```python
from build123d import *

# Parameters (mm, degrees)
BOSS_EXTRUDE1_DEPTH      = 25
BOSS_EXTRUDE1_DEPTH_BACK = 25
SKETCH1_W                = 70
SKETCH1_H                = 10
BOSS_EXTRUDE2_DEPTH      = 10
BOSS_EXTRUDE2_DEPTH_BACK = 10
CUT_EXTRUDE1_DEPTH       = 19
CUT_EXTRUDE1_DEPTH_BACK  = 16
SKETCH3_R                = 3.5


with BuildPart() as part:
    # Sketch1 → Boss-Extrude1 (new, two sides: drawn at the far end of the back side and taken through both)
    with BuildSketch(Plane(origin=(0, 0, 0), x_dir=(1, 0, 0), z_dir=(0, 1, 0)).offset(-BOSS_EXTRUDE1_DEPTH_BACK)):
        Rectangle(SKETCH1_W, SKETCH1_H)
    extrude(amount=BOSS_EXTRUDE1_DEPTH + BOSS_EXTRUDE1_DEPTH_BACK)

    # Sketch2 → Boss-Extrude2 (add, two sides: drawn at the far end of the back side and taken through both)
    with BuildSketch(Plane(origin=(0, 0, 0), x_dir=(1, 0, 0), z_dir=(0, 1, 0)).offset(-BOSS_EXTRUDE2_DEPTH_BACK)):
        with BuildLine():
            Line((-75, 5), (-35, 5))
            Line((-35, 5), (-35, -5))
            Line((-35, -5), (-75, -5))
            ThreePointArc((-75, -5), (-80, 0), (-75, 5))
        make_face()
    extrude(amount=BOSS_EXTRUDE2_DEPTH + BOSS_EXTRUDE2_DEPTH_BACK)

    # Sketch3 → Cut-Extrude1 (cut, two sides: drawn at the far end of the back side and taken through both)
    with BuildSketch(Plane(origin=(0, 0, 0), x_dir=(1, 0, 0), z_dir=(0, 1, 0)).offset(-CUT_EXTRUDE1_DEPTH_BACK)):
        with Locations(Location((-75.333177097, 0, 0), (0, 0, 270))):
            Circle(SKETCH3_R)
        with Locations(Location((-55, 0, 0), (0, 0, 270))):
            Circle(SKETCH3_R)
    extrude(amount=CUT_EXTRUDE1_DEPTH + CUT_EXTRUDE1_DEPTH_BACK, mode=Mode.SUBTRACT)


solid = part.part
```
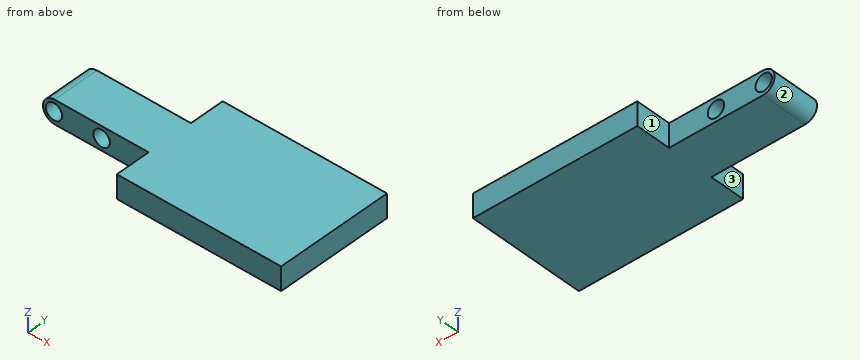
CAD build for the part. Positions are in the model's coordinates, mm. Face numbers are marked on the shaded views. A direction names the side the tool comes from. Round coordinates to 2 decimals unless told otherwise and drop trailing zeros. Order: outer loops, then holes, each group sorted by start corner. A loop starts at its lowest first (then second) coordinate and runs counter-clockwise, first axis right, second up. Notation, with made-up numbers: (86.25, -2.75) -> (121.25, -2.75) arc R19 cw to (121.25, 34.25) -> close; hole circle Ø5 at (62.5, 74). An arc over 180 degrees is marked (long way). Write item = value, one per line.
(1) 3-axis set-ups, long thin cutter, end or side, ignore diameter. For the marked faces 1, 2 and 3: which of +Z, -Z, +X, -X, +Y, -Y reach the whole face in a straight line?
Answers follow:
face_1 = +Z, -Z, -X, +Y
face_2 = -X, +Y, -Y
face_3 = +Z, -Z, -X, -Y
(2) Cut at C-C (y = 6). Write the cut outline in (x, z), plus the area to 3 significant figures.
Answers follow:
outline = (-75, -5) -> (35, -5) -> (35, 5) -> (-75, 5) arc R5 ccw to start; hole circle Ø7 at (-75.33, 0); hole circle Ø7 at (-55, 0)
area = 1,060 mm²
(3) Drill centre lines: L1, parallel to X at y = -2, z = 0; L2, parallel to Z at x = -55, y = -4; L3, parallel to X at y = 7, z = 2.25. Where is each one in solid material? Low to high.
Answers follow:
L1 = -80 to -78.83, -71.83 to -58.5, -51.5 to 35
L2 = -5 to -3.5, 3.5 to 5
L3 = -79.47 to -78.01, -72.65 to -57.68, -52.32 to 35
(4) Flat gauge pins, fed straight in: P1, Ø3, axis at x = -46.5, z = -0.5, coming from the +Y side; P2, Ø3, axis at y = -1.5, z = 2, coming from the -X side. Where does each tip first touch, or does it go through?
Answers follow:
P1 = 10
P2 = -79.97
(5) Cut at B-B (z = 0). Write the cut outline in (x, y), plus the area to 3 significant figures.
Answers follow:
outline = (-80, -10) -> (-78.83, -10) -> (-78.83, 10) -> (-80, 10) -> close; (-71.83, -10) -> (-58.5, -10) -> (-58.5, 10) -> (-71.83, 10) -> close; (-51.5, -10) -> (-35, -10) -> (-35, -25) -> (35, -25) -> (35, 25) -> (-35, 25) -> (-35, 10) -> (-51.5, 10) -> close
area = 4,120 mm²
(6) Cut at A-A (x = -55). Write the cut outline in (y, z), plus the area to 3 significant figures.
Answers follow:
outline = (-10, -5) -> (10, -5) -> (10, -3.5) -> (-10, -3.5) -> close; (-10, 3.5) -> (10, 3.5) -> (10, 5) -> (-10, 5) -> close
area = 60.0 mm²
(7) Cut at D-D (x = -69). Write the cut outline in (y, z).
Answers follow:
outline = (-10, -5) -> (10, -5) -> (10, 5) -> (-10, 5) -> close
